Verification items for the finished model (mm, model axes). A direction names the side the tool comes from. Coordinates: 2 decimals unless noted, no trailing zeros. Write each loop counter-clockwise with the first axis right and the second up, starting at its lowest first coordinate (ties: lowest second). Pieces come first, ordered by that corner, then holes. Notation, with made-up numbers: (22.5, 45.25) - (48.5, 45.25) arc R23 ccw to (48.5, 79.25) - close; hole circle Ø1 at (40.25, 32). An arc over 180 degrees is marked (long way). Answer as CSV lines item,"result". Start each with the question number.
Autodesk Inventor part; units mm, degrees
ref_plane "YZ Plane" through (0, 0, 0) normal (1, 0, 0) x (0, 1, 0)
ref_plane "XZ Plane" through (0, 0, 0) normal (0, 1, 0) x (-1, 0, 0)
ref_plane "XY Plane" through (0, 0, 0) normal (0, 0, 1) x (1, 0, 0)
sketch "Sketch1" plane through (0, 0, 0) normal (0, 1, 0) x (-1, 0, 0)
  line L0 (22.4663, 31.1531) -> (-22.4663, 31.1531)
  line L1 (-22.4663, 31.1531) -> (-22.4663, -31.1531)
  line L2 (-22.4663, -31.1531) -> (22.4663, -31.1531)
  line L3 (22.4663, -31.1531) -> (22.4663, 31.1531)
  point P0 (0, 0)
  point P1 (22.4663, 0)
  point P2 (0, -31.1531)
  dimension "d0" = 62.3062
  dimension "d1" = 44.9326
extrude "Extrusion1" add sketch "Sketch1" along normal blind 0.5334
sketch "Sketch2" plane through (0, 0.5334, 0) normal (0, 1, 0) x (1, 0, 0)
  line L0 (22.4663, -31.1531) -> (22.4663, 31.1531)
  line L1 (-22.4663, 31.1531) -> (22.4663, 31.1531)
  line L2 (22.4663, 31.1531) -> (22.4663, 29.9085)
  line L3 (22.4663, 29.9085) -> (-22.4663, 29.9085)
  line L4 (-22.4663, 29.9085) -> (-22.4663, 31.1531)
  line L5 (-22.4663, -31.1531) -> (22.4663, -31.1531)
  line L6 (22.4663, -31.1531) -> (22.4663, -29.9085)
  line L7 (22.4663, -29.9085) -> (-22.4663, -29.9085)
  line L8 (-22.4663, -29.9085) -> (-22.4663, -31.1531)
  line L9 (-22.4663, -31.1531) -> (22.4663, -31.1531)
  point P0 (0, 0)
  dimension "d4" = 1.2446
  dimension "d5" = 1.2446
  dimension "d6" = 59.817
  dimension "d7" = 0
extrude "Extrusion2" add sketch "Sketch2" along normal blind 2.54
sketch "Sketch3" plane through (0, 0.5334, 0) normal (0, 1, 0) x (1, 0, 0)
  line L0 (22.4663, 29.9085) -> (-22.4663, 29.9085)
  line L1 (4.9276, 29.9085) -> (-4.9276, 29.9085)
  line L2 (-4.9276, 29.9085) -> (-4.9276, 22.6949)
  line L3 (0, 17.7673) -> (0, 17.7673)
  line L4 (4.9276, 22.6949) -> (4.9276, 29.9085)
  arc A0 (-4.9276, 22.6949) -> (0, 17.7673) centre (0, 22.6949) ccw
  arc A1 (0, 17.7673) -> (4.9276, 22.6949) centre (0, 22.6949) ccw
  line L5 (22.4663, -29.9085) -> (-22.4663, -29.9085)
  line L6 (4.9276, -29.9085) -> (-4.9276, -29.9085)
  line L7 (-4.9276, -29.9085) -> (-4.9276, -22.6949)
  line L8 (0, -17.7673) -> (0, -17.7673)
  line L9 (4.9276, -22.6949) -> (4.9276, -29.9085)
  arc A2 (4.9276, -22.6949) -> (0, -17.7673) centre (0, -22.6949) ccw
  arc A3 (0, -17.7673) -> (-4.9276, -22.6949) centre (0, -22.6949) ccw
  point P0 (0, 0)
  point P1 (-4.9276, 17.7673)
  point P2 (4.9276, 17.7673)
  point P3 (0, 17.7673)
  point P4 (-4.9276, -17.7673)
  point P5 (4.9276, -17.7673)
  dimension "d10" = 12.1412
  dimension "d11" = 9.8552
  dimension "d12" = 4.9276
  dimension "d13" = 9.8552
  dimension "d14" = 12.1412
  dimension "d15" = 4.9276
  dimension "d16" = 4.9276
extrude "Extrusion3" add sketch "Sketch3" along normal blind 4.826
sketch "Sketch4" plane through (0, 3.0734, 0) normal (0, 1, 0) x (1, 0, 0)
  line L0 (-22.4663, -31.1531) -> (22.4663, -31.1531)
  line L1 (4.9276, -29.9085) -> (-4.9276, -29.9085)
  line L2 (-4.9276, -29.9085) -> (-4.9276, -31.1531)
  line L3 (-4.9276, -31.1531) -> (4.9276, -31.1531)
  line L4 (4.9276, -31.1531) -> (4.9276, -29.9085)
  line L5 (22.4663, 31.1531) -> (-22.4663, 31.1531)
  line L6 (4.9276, 29.9085) -> (-4.9276, 29.9085)
  line L7 (-4.9276, 29.9085) -> (-4.9276, 31.1531)
  line L8 (-4.9276, 31.1531) -> (4.9276, 31.1531)
  line L9 (4.9276, 31.1531) -> (4.9276, 29.9085)
  point P0 (0, 0)
extrude "Extrusion4" add sketch "Sketch4" along normal blind 2.286
chamfer "Chamfer1" distance 1.2446 angle 45 2 edges at (0, 5.3594, 31.1531) (0, 5.3594, -31.1531)
sketch "Sketch5" plane through (0, 0, 0) normal (0, -1, 0) x (1, 0, 0)
  line L0 (22.4663, -31.1531) -> (-22.4663, -31.1531)
  line L1 (-3.8481, -31.1531) -> (3.8481, -31.1531)
  line L2 (3.8481, -31.1531) -> (3.8481, -28.1813)
  line L3 (3.8481, -28.1813) -> (-3.8481, -28.1813)
  line L4 (-3.8481, -28.1813) -> (-3.8481, -31.1531)
  line L5 (-22.4663, 31.1531) -> (22.4663, 31.1531)
  line L6 (-3.8481, 31.1531) -> (3.8481, 31.1531)
  line L7 (3.8481, 31.1531) -> (3.8481, 28.1813)
  line L8 (3.8481, 28.1813) -> (-3.8481, 28.1813)
  line L9 (-3.8481, 28.1813) -> (-3.8481, 31.1531)
  point P0 (0, 0)
  point P1 (0, -31.1531)
  point P2 (0, -28.1813)
  point P3 (0, 28.1813)
  point P4 (0, 31.1531)
  dimension "d24" = 7.6962
  dimension "d25" = 2.9718
  dimension "d26" = 2.9718
extrude "Extrusion5" cut sketch "Sketch5" against normal blind 3.6068
sketch "Sketch6" plane through (0, 5.3594, 0) normal (0, 1, 0) x (1, 0, 0)
  line L0 (0, 19.9009) -> (0, 19.9009)
  line L1 (2.0955, 21.9964) -> (2.0955, 24.765)
  line L2 (0, 26.8605) -> (0, 26.8605)
  line L3 (-2.0955, 24.765) -> (-2.0955, 21.9964)
  line L4 (4.9276, 31.1531) -> (-4.9276, 31.1531)
  arc A0 (0, 19.9009) -> (2.0955, 21.9964) centre (0, 21.9964) ccw
  arc A1 (-2.0955, 21.9964) -> (0, 19.9009) centre (0, 21.9964) ccw
  arc A2 (0, 26.8605) -> (-2.0955, 24.765) centre (0, 24.765) ccw
  arc A3 (2.0955, 24.765) -> (0, 26.8605) centre (0, 24.765) ccw
  circle A4 centre (0, -23.5331) radius 2.2606
  line L5 (-4.9276, -31.1531) -> (4.9276, -31.1531)
  point P0 (0, 0)
  point P1 (2.0955, 26.8605)
  point P2 (2.0955, 19.9009)
  point P3 (-2.0955, 26.8605)
  point P4 (0, 19.9009)
  dimension "d29" = 4.191
  dimension "d30" = 6.9596
  dimension "d31" = 4.2926
  dimension "d32" = 2.0955
  dimension "d33" = 2.0955
  dimension "d34" = 2.0955
  dimension "d35" = 7.62
  dimension "d38" = 4.5212
extrude "Extrusion6" cut sketch "Sketch6" against normal through all
properties part number "SSR-40 DA BOTTOM" material "Nickel-Copper Alloy 400"
1. Access from +Z, -Z, +X, -X, +Y, -Y to the whole of each face (thin tool, end or side, straight path). Record for faces 4 (the face through (0.05, 2.72, -26.86)), 5 (the face through (3.848, 2, 30)), 6 (the face through (14, 3.073, -31)), 7 (the face through (3.848, 2, -30)).
2. Cross-section at D-D (z = -3.5). Record the cut outline in (x, y), and give its area (3 significant figures).
3. Cross-section at C-C (x = -14). Record the cut outline in (y, z).
4. Draft check along X on faces 1 (the face through (0, 3.607, -30)), 2 (the face through (-14, 2, 29.908)), 3 (the face through (-0.11, 2.91, 17.77)). Enter one of: pulls with the +X half, pulls with the -X half, needs draft (parallel to the pull), parting line crosses it, or undercut.
5. Cross-section at B-B (y = 2.4). Count the separate pieces of the cut face and the enclosed holes in it, and give its area (3 significant figures).
6. Scan lines: line 1 along Z through (x, y) = (0, 3.1); line 2 along Z through (x, y) = (0, 4.2); line 3 along Z through (x, y) = (12.5, 2.2). Record each from-to range of solid material in increasing order. Write a range as from..to.
7. Cross-section at A-A (x = 0). Record the cut outline in (y, z), and give its area (3 significant figures).
8. Depth check by flat-ended pin: P1, Ø1, axis at x = -13.5, z = 30.5, coming from the +Y side; P2, Ø2.5, axis at y = 3.5, z = -25.5, coming from the +X side; P3, Ø3, axis at y = 3.5, z = 18.5, coming from the -X side; P4, Ø2.5, axis at x = 0, z = 23.53, coming from the -Y side. Enter the tip coordinate at first touch or a pass-through.
Completed:
1,face 4,"+Y, -Y"
1,face 5,"+Z, -Y"
1,face 6,"+Z, -Z, +X, +Y"
1,face 7,"-Z, -Y"
2,outline,"(-22.47, 0) - (22.47, 0) - (22.47, 0.53) - (-22.47, 0.53) - close"
2,area,"24.0 mm2"
3,outline,"(0, -31.15) - (3.07, -31.15) - (3.07, -29.91) - (0.53, -29.91) - (0.53, 29.91) - (3.07, 29.91) - (3.07, 31.15) - (0, 31.15) - close"
4,face 1,"undercut"
4,face 2,"needs draft"
4,face 3,"parting line crosses it"
5,separate pieces,"2"
5,enclosed holes,"2"
5,area,"243 mm2"
6,line 1,"z = -28.18..-26.86, -19.9..-17.77, 17.77..21.27, 25.79..28.18"
6,line 2,"z = -31.07..-26.86, -19.9..-17.77, 17.77..21.27, 25.79..31.07"
6,line 3,"z = -31.15..-29.91, 29.91..31.15"
7,outline,"(0, -28.18) - (3.61, -28.18) - (3.61, -31.15) - (4.11, -31.15) - (5.36, -29.91) - (5.36, -26.86) - (0, -26.86) - close; (0, -19.9) - (5.36, -19.9) - (5.36, -17.77) - (0.53, -17.77) - (0.53, 17.77) - (5.36, 17.77) - (5.36, 21.27) - (0, 21.27) - close; (0, 25.79) - (5.36, 25.79) - (5.36, 29.91) - (4.11, 31.15) - (3.61, 31.15) - (3.61, 28.18) - (0, 28.18) - close"
7,area,"77.9 mm2"
8,P1,"stops at y = 3.07"
8,P2,"stops at x = 4.93"
8,P3,"stops at x = -4.13"
8,P4,"passes through"
